from build123d import *

# Parameters (mm, degrees)
BASE_W                   = 600
BASE_H                   = 400
EXTRUDE_1_DEPTH          = 120
SKETCH_5_W               = 600
SKETCH_5_H               = 10
SKETCH_5_H_2             = 5
EXTRUDE_4_DEPTH          = 20
SKETCH_6_W               = 30
SKETCH_6_H               = 155
EXTRUDE_5_DEPTH          = 20
SKETCH_7_W               = 560
SKETCH_7_H               = 110
CUT_EXTRUDE_1_DEPTH      = 732.0266753
CUT_EXTRUDE_2_DEPTH      = 565
CUT_EXTRUDE_2_DEPTH_BACK = 5
SKETCH_8_R               = 2.5
CUT_EXTRUDE_3_DEPTH      = 715.702735408
CUT_EXTRUDE_3_DEPTH_BACK = 715.702735408
SKETCH_9_W               = 40
SKETCH_9_H               = 20
SKETCH_10_W              = 100
SKETCH_10_H              = 100
CUT_EXTRUDE_4_DEPTH      = 1
CUT_EXTRUDE_5_DEPTH      = 567
CUT_EXTRUDE_5_DEPTH_BACK = 7
SKETCH_11_W              = 400
SKETCH_11_H              = 1
CUT_EXTRUDE_7_DEPTH      = 567
CUT_EXTRUDE_7_DEPTH_BACK = 7
SKETCH_13_W              = 1
SKETCH_13_H              = 80
SKETCH_13_W_2            = 2
SKETCH_15_W              = 10
SKETCH_15_H              = 39.5
EXTRUDE_7_DEPTH          = 561


with BuildPart() as part:
    # base → 凸台-拉伸1 (new body)
    with BuildSketch(Plane(origin=(0, 0, 0), x_dir=(1, 0, 0), z_dir=(0, 1, 0))):
        with Locations((300, -200)):
            Rectangle(BASE_W, BASE_H)
    extrude(amount=EXTRUDE_1_DEPTH)

    # 草图5 → 凸台-拉伸4 (add)
    with BuildSketch(Plane.XZ):
        with Locations((300, 150)):
            Rectangle(SKETCH_5_W, SKETCH_5_H)
        with Locations((300, 100)):
            Rectangle(SKETCH_5_W, SKETCH_5_H)
        with Locations((300, 2.5)):
            Rectangle(SKETCH_5_W, SKETCH_5_H_2)
        with Locations((300, 50)):
            Rectangle(SKETCH_5_W, SKETCH_5_H)
        with Locations((300, 250)):
            Rectangle(SKETCH_5_W, SKETCH_5_H)
        with Locations((300, 200)):
            Rectangle(SKETCH_5_W, SKETCH_5_H)
        with Locations((300, 300)):
            Rectangle(SKETCH_5_W, SKETCH_5_H)
        with Locations((300, 350)):
            Rectangle(SKETCH_5_W, SKETCH_5_H)
        with Locations((300, 397.5)):
            Rectangle(SKETCH_5_W, SKETCH_5_H_2)
    extrude(amount=EXTRUDE_4_DEPTH)

    # 草图6 → 凸台-拉伸5 (add)
    with BuildSketch(Plane.XZ):
        with Locations((15, 322.5)):
            Rectangle(SKETCH_6_W, SKETCH_6_H)
        with Locations((15, 77.5)):
            Rectangle(SKETCH_6_W, SKETCH_6_H)
        with Locations((585, 322.5)):
            Rectangle(SKETCH_6_W, SKETCH_6_H)
        with Locations((585, 77.5)):
            Rectangle(SKETCH_6_W, SKETCH_6_H)
    extrude(amount=EXTRUDE_5_DEPTH)

    # 草图7 → 切除-拉伸1 (cut, through all)
    with BuildSketch(Plane.XY.offset(400)):
        with Locations((300, 65)):
            Rectangle(SKETCH_7_W, SKETCH_7_H)
    extrude(amount=-CUT_EXTRUDE_1_DEPTH, mode=Mode.SUBTRACT)

    # 草图8 → 切除-拉伸2 (cut, two sides: drawn at the far end of the back side and taken through both)
    with BuildSketch(Plane(origin=(20, 0, 0), x_dir=(0, 0, -1), z_dir=(1, 0, 0)).offset(-CUT_EXTRUDE_2_DEPTH_BACK)):
        with Locations(Location((-360, 90, 0), (0, 0, 90))):
            Circle(SKETCH_8_R)
        with Locations(Location((-60, 90, 0), (0, 0, 90))):
            Circle(SKETCH_8_R)
        with Locations(Location((-340, 70, 0), (0, 0, 90))):
            Circle(SKETCH_8_R)
        with Locations(Location((-360, 70, 0), (0, 0, 90))):
            Circle(SKETCH_8_R)
        with Locations(Location((-340, 90, 0), (0, 0, 90))):
            Circle(SKETCH_8_R)
        with Locations(Location((-60, 70, 0), (0, 0, 90))):
            Circle(SKETCH_8_R)
        with Locations(Location((-40, 70, 0), (0, 0, 90))):
            Circle(SKETCH_8_R)
        with Locations(Location((-40, 90, 0), (0, 0, 90))):
            Circle(SKETCH_8_R)
        with Locations(Location((-350, 80, 0), (0, 0, 90))):
            Circle(SKETCH_8_R)
        with Locations(Location((-50, 80, 0), (0, 0, 90))):
            Circle(SKETCH_8_R)
    extrude(amount=CUT_EXTRUDE_2_DEPTH + CUT_EXTRUDE_2_DEPTH_BACK, mode=Mode.SUBTRACT)

    # 草图9 → 切除-拉伸3 (cut, two sides: drawn at the far end of the back side and taken through both)
    with BuildSketch(Plane(origin=(20, 0, 0), x_dir=(0, 0, -1), z_dir=(1, 0, 0)).offset(-CUT_EXTRUDE_3_DEPTH_BACK)):
        with Locations((-350, 30)):
            Rectangle(SKETCH_9_W, SKETCH_9_H)
        with Locations((-50, 30)):
            Rectangle(SKETCH_9_W, SKETCH_9_H)
    extrude(amount=CUT_EXTRUDE_3_DEPTH + CUT_EXTRUDE_3_DEPTH_BACK, mode=Mode.SUBTRACT)

    # 草图10 → 切除-拉伸4 (cut)
    with BuildSketch(Plane(origin=(0, 10, 0), x_dir=(1, 0, 0), z_dir=(0, 1, 0))):
        with Locations((300, -200)):
            Rectangle(SKETCH_10_W, SKETCH_10_H)
    extrude(amount=-CUT_EXTRUDE_4_DEPTH, mode=Mode.SUBTRACT)

    # 草图11 → 切除-拉伸5 (cut, two sides: drawn at the far end of the back side and taken through both)
    with BuildSketch(Plane.ZY.offset(-580).offset(-CUT_EXTRUDE_5_DEPTH_BACK)):
        with Locations((200, 80)):
            Rectangle(SKETCH_11_W, SKETCH_11_H)
    extrude(amount=CUT_EXTRUDE_5_DEPTH + CUT_EXTRUDE_5_DEPTH_BACK, mode=Mode.SUBTRACT)

    # 草图13 → 切除-拉伸7 (cut, two sides: drawn at the far end of the back side and taken through both)
    with BuildSketch(Plane.ZY.offset(-580).offset(-CUT_EXTRUDE_7_DEPTH_BACK)):
        with Locations((50, 80)):
            Rectangle(SKETCH_13_W, SKETCH_13_H)
        with Locations((350, 80)):
            Rectangle(SKETCH_13_W_2, SKETCH_13_H)
    extrude(amount=CUT_EXTRUDE_7_DEPTH + CUT_EXTRUDE_7_DEPTH_BACK, mode=Mode.SUBTRACT)

    # 草图15 → 凸台-拉伸7 (add)
    with BuildSketch(Plane(origin=(20, 0, 0), x_dir=(0, 0, -1), z_dir=(1, 0, 0))):
        with Locations((-395, 100.25)):
            Rectangle(SKETCH_15_W, SKETCH_15_H)
        with Locations((-5, 100.25)):
            Rectangle(SKETCH_15_W, SKETCH_15_H)
    extrude(amount=EXTRUDE_7_DEPTH)


solid = part.part
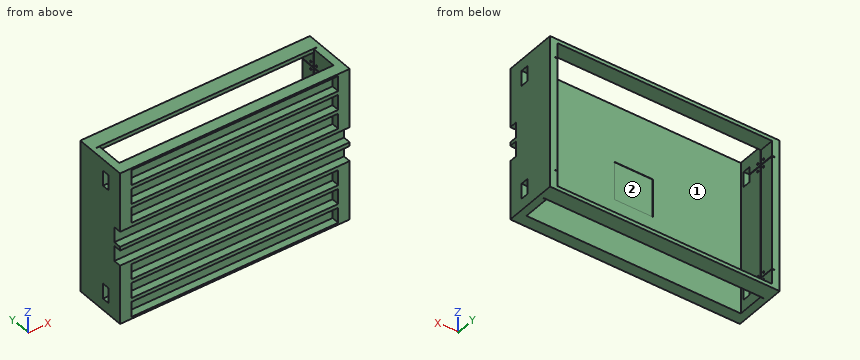
CAD build for the part. Positions are in the model's coordinates, mm. Face numbers are marked on the shaded views. Round coordinates to 2 decimals unless told otherwise and drop trailing zeros. Write each loop counter-clockwise with the first axis right and the second up, starting at its lowest first coordinate (ties: lowest second). Pieces come first, ordered by that corner, then holes.
(1) Probe line 1 along Y through (x, z) = (583, 60); line 2 along X through (y, z) = (99.5, 325); line 3 along Z through (x, y) = (562, 114). List the from-to ranges inside material, lowest first.
(2) Slice it at B-B, the plane y = 30. Write the cut outline in (x, z).
(3) Slice it at D-D, the plane x = 231. Count the separate pieces of the cut face and the enclosed holes in it, and give its area (3 significant figures).
(4) Mould opens along Z. For the marked faces 1 and 2 say: pulls with the +Z half, pulls with the -Z half, needs draft (parallel to the pull), parting line crosses it, or undercut.
(5) Slice it at C-C, the plane z = 134. Write the cut outline in (x, y).
(6) Slice it at A-A, the plane y = 58. Write the cut outline in (x, z), and give its area (3 significant figures).
(7) Drop flat-ended pins along their axis: P1, Ø22, axis at x = 317.5, y = -8.5, coming from the -Z side; P2, Ø12, axis at x = 244.5, z = 65.5, coming from the +Y side. Give the stop position or say it passes through.
From the geometry:
1. line 1: y = -20 to 20, 40 to 67.5, 72.5 to 79.5, 80.5 to 87.5, 92.5 to 120
1. line 2: x = 0 to 20, 580 to 600
1. line 3: z = 0 to 10, 390 to 400
2. outline: (0, 0) - (20, 0) - (20, 30) - (0, 30) - close; (0, 70) - (20, 70) - (20, 330) - (0, 330) - close; (0, 370) - (20, 370) - (20, 400) - (0, 400) - close; (580, 0) - (600, 0) - (600, 30) - (580, 30) - close; (580, 70) - (600, 70) - (600, 330) - (580, 330) - close; (580, 370) - (600, 370) - (600, 400) - (580, 400) - close
3. separate pieces: 3
3. enclosed holes: 0
3. area: 6,390 mm2
4. face 1: needs draft
4. face 2: undercut
5. outline: (0, -20) - (30, -20) - (30, 0) - (570, 0) - (570, -20) - (600, -20) - (600, 120) - (580, 120) - (580, 80.5) - (587, 80.5) - (587, 79.5) - (580, 79.5) - (580, 10) - (20, 10) - (20, 79.5) - (13, 79.5) - (13, 80.5) - (20, 80.5) - (20, 120) - (0, 120) - close
6. outline: (0, 0) - (20, 0) - (20, 49.5) - (13, 49.5) - (13, 50.5) - (20, 50.5) - (20, 349) - (13, 349) - (13, 351) - (20, 351) - (20, 400) - (0, 400) - close; (580, 0) - (600, 0) - (600, 400) - (580, 400) - (580, 351) - (587, 351) - (587, 349) - (580, 349) - (580, 50.5) - (587, 50.5) - (587, 49.5) - (580, 49.5) - close
6. area: 16,000 mm2
7. P1: stops at z = 0
7. P2: stops at y = 10
